Input: part model. Units: mm. Frame: model coordinates. A direction names the side the tool comes from. Give positions to 0.01 mm unless a question says otherwise; leave off trailing zeros. Write each loop counter-clockwise with the first axis right and the second up, starting at its lowest first coordinate (ties: lowest second). Pieces come first, ordered by that corner, then holes. Notation, with made-up numbers: M 37.25,-36.5 L 68.25,-36.5 A12 cw 68.25,-21.5 Z; hole C 21.5,42 d10. An arc over 180 degrees is marked long. Use CSV: the item, a comma, the result in double quotes. Start each with the question number.
Autodesk Inventor part; units mm, degrees
ref_plane "YZ Plane" through (0, 0, 0) normal (1, 0, 0) x (0, 1, 0)
ref_plane "XZ Plane" through (0, 0, 0) normal (0, 1, 0) x (-1, 0, 0)
ref_plane "XY Plane" through (0, 0, 0) normal (0, 0, 1) x (1, 0, 0)
sketch "Sketch1" plane through (0, 0, 0) normal (0, 0, 1) x (1, 0, 0)
  point P0 (0, 0)
sketch "Sketch2" plane through (0, 0, 0) normal (0, 0, 1) x (1, 0, 0)
  line L0 (-15, 113.5) -> (15, 113.5)
  line L1 (15, 113.5) -> (15, 50)
  line L2 (15, 50) -> (-15, 50) construction
  line L3 (-15, 50) -> (-15, 113.5)
  circle A0 centre (0, 0) radius 5 construction
  line L4 (-15, 50) -> (-4.9047, -0.9714)
  line L5 (15, 50) -> (4.9047, -0.9714)
  arc A1 (-4.9047, -0.9714) -> (4.9047, -0.9714) centre (0, 0) ccw
  point P0 (0, 50)
  dimension "d0" = 30
  dimension "d1" = 63.5
  dimension "d2" = 10
  dimension "d3" = 50
extrude "Extrusion1" add sketch "Sketch2" along normal blind 5
sketch "Sketch3" plane through (0, 0, 5) normal (0, 0, 1) x (1, 0, 0)
  line L0 (-10, 108.5) -> (10, 108.5) construction
  line L1 (10, 108.5) -> (10, 55) construction
  line L2 (10, 55) -> (-10, 55) construction
  line L3 (-10, 55) -> (-10, 108.5) construction
  line L4 (15, 113.5) -> (-15, 113.5) construction
  circle A0 centre (-5, 106) radius 2.25
  circle A1 centre (5, 106) radius 2.25
  circle A2 centre (-5, 57.5) radius 2.25
  circle A3 centre (5, 57.5) radius 2.25
  line L5 (-10, 61.5) -> (10, 61.5)
  line L6 (10, 61.5) -> (10, 102)
  line L7 (10, 102) -> (-10, 102)
  line L8 (-10, 102) -> (-10, 61.5)
  line L9 (0, 108.5) -> (0, 55) construction
  point P0 (0, 0)
  point P1 (-10, 81.75)
  point P2 (10, 81.75)
  point P3 (0, 81.75)
  dimension "d6" = 20
  dimension "d7" = 53.5
  dimension "d8" = 5
  dimension "d9" = 4.5
  dimension "d11" = 2.75
  dimension "d12" = 2.5
  dimension "d13" = 2.75
  dimension "d14" = 2.5
  dimension "d15" = 40.5
extrude "Extrusion2" cut sketch "Sketch3" against normal up to next
sketch "Sketch4" plane through (15, 50, 0) normal (1, 0, 0) x (0, 0, -1)
  line L0 (-5, 52) -> (0, 52)
  line L1 (0, 52) -> (0, 11.5)
  line L2 (0, 11.5) -> (-5, 11.5)
  line L3 (-5, 11.5) -> (-5, 52)
  line L4 (-5, 52) -> (0, 52)
  line L5 (-5, 11.5) -> (0, 11.5)
  line L6 (0, 63.5) -> (0, 0)
  point P0 (0, -50)
  point P1 (-2.5, 52)
  point P2 (-2.5, 11.5)
  point P3 (0, 31.75)
extrude "Extrusion3" cut sketch "Sketch4" against normal up to surface (5 mm away)
sketch "Sketch8" plane through (0, 0, 0) normal (0, 0, -1) x (-1, 0, 0)
  line L0 (15, 102) -> (10, 102)
  line L1 (10, 102) -> (10, 61.5)
  line L2 (10, 61.5) -> (15, 61.5)
  line L3 (15, 61.5) -> (15, 102)
  line L4 (15, 50) -> (15, 113.5)
  line L5 (10, 102) -> (10, 61.5)
  point P0 (0, 0)
  point P1 (15, 81.75)
  point P2 (10, 81.75)
  point P3 (12.5, 61.5)
  point P4 (12.5, 102)
extrude "Extrusion6" add sketch "Sketch8" along normal blind 27.5
sketch "Sketch9" plane through (-10, 61.5, 5) normal (1, 0, 0) x (0, 0, -1)
  line L0 (27.5, 40.5) -> (32.5, 40.5)
  line L1 (32.5, 40.5) -> (32.5, 0)
  line L2 (32.5, 0) -> (27.5, 0)
  line L3 (27.5, 0) -> (27.5, 40.5)
  line L4 (32.5, 40.5) -> (32.5, 0)
  line L5 (5, 40.5) -> (32.5, 40.5)
  line L6 (5, 0) -> (32.5, 0)
  point P0 (5, -61.5)
  point P1 (32.5, 20.25)
  point P2 (30, 40.5)
  point P3 (30, 0)
  dimension "d27" = 5
extrude "Extrusion7" add sketch "Sketch9" along normal blind 20
equation "\"d0\" = s_depth + 2 * b_mat_thickness"
equation "\"d1\" = 2 * s_land + s_width + 2 * b_mat_thickness"
equation "\"d4\" = b_mat_thickness"
equation "\"d6\" = s_depth"
equation "\"d7\" = s_width + 2 * s_land"
equation "\"d8\" = b_mat_thickness"
equation "\"d9\" = s_hole_dia"
equation "\"d11\" = s_hole_side_dist"
equation "\"d12\" = s_hole_front_dist"
equation "\"d13\" = s_hole_side_dist"
equation "\"d14\" = s_hole_front_dist"
equation "\"d15\" = s_width"
equation "\"d16\" = b_mat_thickness"
equation "\"d25\" = -s_land_dist_top + s_height - s_land_thickness"
equation "\"d27\" = b_mat_thickness"
equation "\"d28\" = s_depth"
properties part number "Lower_leg"
Q1. Pull-direction query (X, two-part tool) for faces 1 (the flat face through (10, 82, -25)), 2 (the cylindrical face through (-5.488, 103.804, 2.535)), 3 (the flat face through (3, 102, 3)); classes: released by +X, released by -X, zero draft, split by the parting line, or undercut.
Q2. Material intervals for L1, parallel to X at y = 57, z = 1; L2, parallel to Y at x = -7, z = -24; L3, parallel to Z at x = 2, y = 52, sorted ascending. Write a range as [from, to].
Q3. Section A-A, the plane y = 57.5. Return the cut outline in (x, z), and give its area (3 significant figures).
Q4. Section B-B, the plane x = -1.5. Return the cut outline in (y, z).
Q5. Set-up query: faces 4 (the flat face through (-10, 82, -9)), 5 (the flat face through (0, 81, -22.5)), 6 (the flat face through (0, 36, 0)). Return all of +Z, -Z, +X, -X, +Y, -Y with unobstructed straight access to the full face (end or side cutting, diameter ignored); none if empty.
Q6. First-contact query: pin 1 Ø3.5 at (x, y) = (5, 57.5) entering from -Z; pin 2 Ø7 at (x, y) = (5, 106) entering from -Z; pin 3 Ø7.5 at (x, z) = (-4.5, -20) entering from +Y; pin 4 Ø6 at (x, y) = (0, 74.5) entering from +Z. Flat tips, straight axial feed; report the tip coordinate or a pass-through.
Q7. Section C-C, the plane z = -16.5. Return the cut outline in (x, y).
Q8. Section D-D, the plane y = 88. Return the cut outline in (x, z).
Check result:
1,face 1,"released by +X"
1,face 2,"undercut"
1,face 3,"zero draft"
2,L1,"x = [-15, -7.19], [-2.81, 2.81], [7.19, 15]"
2,L2,"y = [61.5, 102]"
2,L3,"z = [0, 5]"
3,outline,"M -15,0 L -7.25,0 L -7.25,5 L -15,5 Z; M -2.75,0 L 2.75,0 L 2.75,5 L -2.75,5 Z; M 7.25,0 L 15,0 L 15,5 L 7.25,5 Z"
3,area,"105 mm²"
4,outline,"M -4.77,0 L 61.5,0 L 61.5,5 L -4.77,5 Z; M 61.5,-27.5 L 102,-27.5 L 102,-22.5 L 61.5,-22.5 Z; M 102,0 L 113.5,0 L 113.5,5 L 102,5 Z"
5,face 4,"+Z, +X"
5,face 5,"+Z, +X, +Y, -Y"
5,face 6,"-Z, +X, -X, -Y"
6,pin 1,"passes through"
6,pin 2,"stops at z = 0"
6,pin 3,"stops at y = 102"
6,pin 4,"stops at z = -22.5"
7,outline,"M -15,61.5 L -10,61.5 L -10,102 L -15,102 Z"
8,outline,"M -15,-27.5 L 10,-27.5 L 10,-22.5 L -10,-22.5 L -10,5 L -15,5 Z"
